The drawing under review shows one solid part. Ordinate dimensions are in mm from its lowest x, y, z. A direction names the side the tool comes from. Coordinates: 2 decimals unless noted, no trailing zeros. Write each loop counter-clockwise with the first axis right and the second up, starting at its lowest first coordinate (ties: lowest second). Pieces come first, ordered by that corner, then holes.
Q1. Insertion check: pin 1 (1.5 mm diameter, centred on x = 8.5, y = 30, fed in from -Z). The pin has a flat end and moves straight along its axis. Give the tip position at first contact, or say it passes through.
Q2. Take a section at A-A (x = 31.75). State how many separate pieces and enclosed holes the cut face has, and give its area (3 significant figures).
Q3. For probe 1 along X at (y, z) = (18, 55.5); probe 2 along X at (y, z) = (31, 61) (1 decimal), list the stretches that pass through material, from the lowest coordinate up.
Q4. Mouldability with a two-part tool opening along X and no side actions: class the marked faces 1, 2, 3 and 4 as pulls with the +X half, pulls with the -X half, needs draft (parallel to the pull), parting line crosses it, or undercut.
Q5. Take a section at B-B (y = 12.7). Give the boundary of the cut face in (x, z) (1 decimal).
Q6. Take a section at D-D (y = 26). Give the boundary of the cut face in (x, z) (1 decimal).
Q7. Machinability: for the marked faces 5 and 6, which of the approach directions +Z, -Z, +X, -X, +Y, -Y give a long, thin tool a straight path to every point of the face, cutting with its end or side? Answer none if there is none.
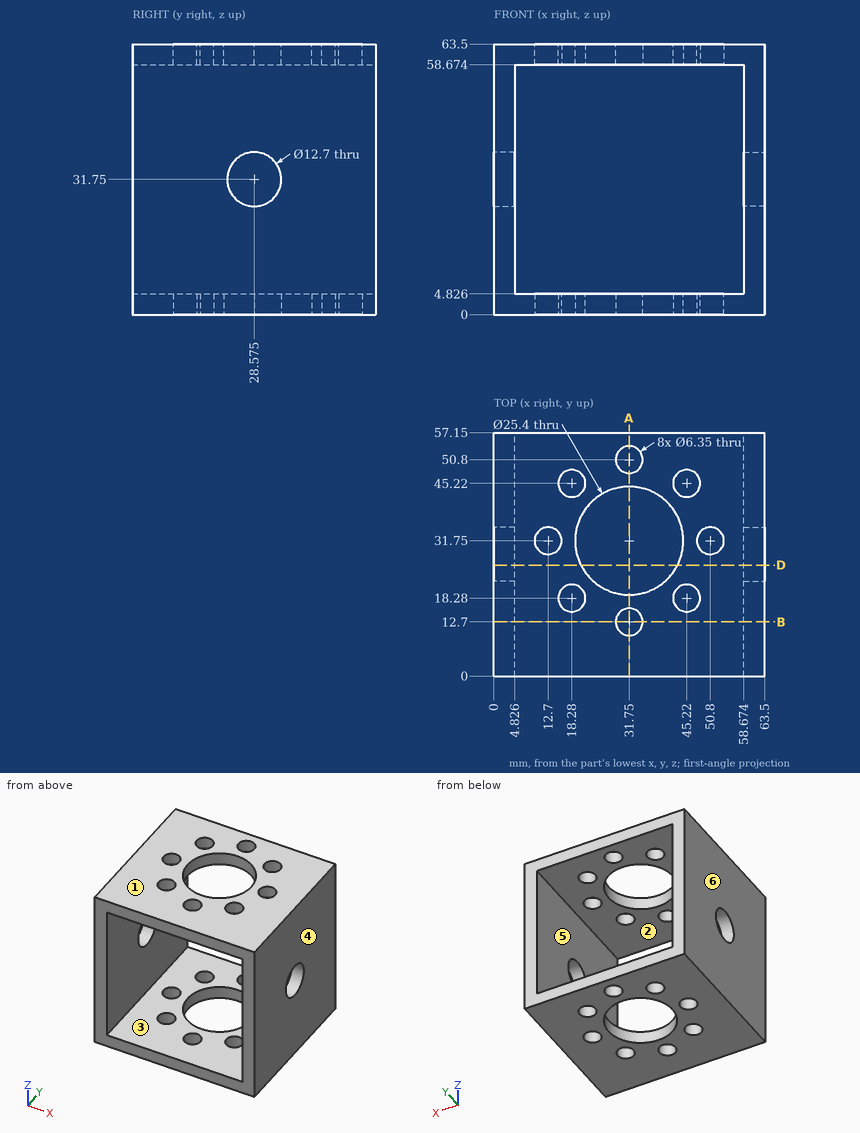
Response:
1. pin 1: stops at z = 0
2. separate pieces: 8
2. enclosed holes: 0
2. area: 184 mm2
3. probe 1: x = 0 to 4.83, 58.67 to 63.5
3. probe 2: x = 0 to 9.6, 15.8 to 19.1, 44.4 to 47.7, 53.9 to 63.5
4. face 1: needs draft
4. face 2: undercut
4. face 3: undercut
4. face 4: pulls with the +X half
5. outline: (0, 0) - (28.6, 0) - (28.6, 4.8) - (4.8, 4.8) - (4.8, 58.7) - (28.6, 58.7) - (28.6, 63.5) - (0, 63.5) - close; (34.9, 0) - (63.5, 0) - (63.5, 63.5) - (34.9, 63.5) - (34.9, 58.7) - (58.7, 58.7) - (58.7, 4.8) - (34.9, 4.8) - close
6. outline: (0, 0) - (20.4, 0) - (20.4, 4.8) - (4.8, 4.8) - (4.8, 25.9) - (0, 25.9) - close; (0, 37.6) - (4.8, 37.6) - (4.8, 58.7) - (20.4, 58.7) - (20.4, 63.5) - (0, 63.5) - close; (43.1, 0) - (63.5, 0) - (63.5, 25.9) - (58.7, 25.9) - (58.7, 4.8) - (43.1, 4.8) - close; (43.1, 58.7) - (58.7, 58.7) - (58.7, 37.6) - (63.5, 37.6) - (63.5, 63.5) - (43.1, 63.5) - close
7. face 5: +Y, -Y
7. face 6: +Z, -Z, -X, +Y, -Y
